Geometry check sheet. Reference: the model listing, model coordinates, mm. A direction names the side the tool comes from. Round coordinates to 2 decimals unless told otherwise and drop trailing zeros. Write each loop counter-clockwise with the first axis right and the second up, starting at its lowest first coordinate (ties: lowest second). Pieces come first, ordered by that corner, then holes.
Item 1: Cross-section at B-B (y = 50). Enter the section's corners in (x, z), then the cut area to 3 significant figures.
Item 2: Draft check along Y on faces 5 (the face through (-21, 0, 0)), 6 (the face through (3.5, 173, 6)), 7 (the face through (-16, 85, 6)), 8 (the face through (21.3, 2.85, 0.92)). Enter one of: pulls with the +Y half, pulls with the -Y half, needs draft (parallel to the pull), parting line crosses it, or undercut.
Item 3: Scan lines: probe 1 along Y at (x, z) = (-19.5, 0); probe 2 along Z at (x, y) = (-20.25, 25); probe 3 along Y at (x, z) = (22.25, 0). Record each from-to range of solid material in increasing order.
Item 4: Cross-section at A-A (y = 7). Enter the section's corners in (x, z).
Item 5: Access from +Z, -Z, +X, -X, +Y, -Y to the whole of each face (thin tool, end or side, straight path). Record for faces 1 (the face through (-17.6, 20, 0)), 2 (the face through (-21, 40, -4)), 3 (the face through (-0.751, 249.86, 3.615)), 4 (the face through (16, 85, 6)).
Item 6: Cross-section at C-C (x = 0). Enter the section's corners in (y, z).
Item 7: Cross-section at D-D (y = 224.5). Enter the section's corners in (x, z), then the cut area to 3 significant figures.
Item 8: Depth check by flat-ended pin: P1, Ø7.5, axis at y = 7, z = 0, coming from the +X side; P2, Ø2, axis at y = 219, z = 6, coming from the -X side; P3, Ø9, axis at x = 6, z = 7, coming from the -Y side; P4, Ø6, axis at x = 23, z = 0, coming from the +Y side. Enter the tip coordinate at first touch or a pass-through.
from build123d import *

# Parameters (mm, degrees)
BOSS_EXTRUDE4_DEPTH     = 10
CUT_EXTRUDE2_DEPTH      = 262.400095639
CUT_EXTRUDE2_DEPTH_BACK = 262.400095639
SKETCH7_R               = 4.25
CUT_EXTRUDE4_DEPTH      = 262.400095639
CUT_EXTRUDE4_DEPTH_BACK = 262.400095639
SKETCH11_W              = 18.643899753
SKETCH11_H              = 220
CUT_EXTRUDE5_DEPTH      = 262.400095639
CUT_EXTRUDE5_DEPTH_BACK = 20
SKETCH12_R              = 2.5
FILLET3_R               = 3


with BuildPart() as part:
    # Sketch6 → Boss-Extrude4 (new, symmetric)
    with BuildSketch(Plane.XY):
        Polygon((-25.1, 0), (-17.6, 0), (-17.6, 40), (-22.1, 40), (-22.1, 80), (22.1, 80), (22.1, 40), (17.6, 40), (17.6, 0), (25.1, 0), (25.1, 85), (3.5, 85), (3.5, 260), (-3.5, 260), (-3.5, 85), (-25.1, 85), align=None)
    extrude(amount=BOSS_EXTRUDE4_DEPTH, both=True)

    # Sketch7 → Cut-Extrude2 (cut, two sides: drawn at the far end of the back side and taken through both)
    with BuildSketch(Plane(origin=(0, 0, 0), x_dir=(0, 0, -1), z_dir=(1, 0, 0)).offset(-CUT_EXTRUDE2_DEPTH_BACK)):
        with Locations((0, 7)):
            Circle(SKETCH7_R)
        with Locations((0, 25)):
            Circle(SKETCH7_R)
    extrude(amount=CUT_EXTRUDE2_DEPTH + CUT_EXTRUDE2_DEPTH_BACK, mode=Mode.SUBTRACT)

    # Sketch11 → Cut-Extrude4 (cut, two sides: drawn at the far end of the back side and taken through both)
    with BuildSketch(Plane(origin=(0, 0, 0), x_dir=(0, 0, -1), z_dir=(1, 0, 0)).offset(-CUT_EXTRUDE4_DEPTH_BACK)):
        with Locations((7.321949876, 150)):
            Rectangle(SKETCH11_W, SKETCH11_H)
    extrude(amount=CUT_EXTRUDE4_DEPTH + CUT_EXTRUDE4_DEPTH_BACK, mode=Mode.SUBTRACT)

    # Sketch12 → Cut-Extrude5 (cut, two sides: drawn at the far end of the back side and taken through both)
    with BuildSketch(Plane(origin=(0, 260, 0), x_dir=(1, 0, 0), z_dir=(0, 1, 0)).offset(-CUT_EXTRUDE5_DEPTH_BACK)):
        with Locations(Location((0, -6, 0), (0, 0, 90))):
            Circle(SKETCH12_R)
    extrude(amount=CUT_EXTRUDE5_DEPTH + CUT_EXTRUDE5_DEPTH_BACK, mode=Mode.SUBTRACT)

    # Fillet3
    fillet3_edges = [part.edges().sort_by_distance(p)[0] for p in [
        (-23.6, 40, 2),
        (23.6, 40, 2),
        (22.1, 40, 6),
        (22.1, 80, 6),
        (-22.1, 80, 6),
        (-22.1, 40, 6),
        (-3.5, 85, 6),
        (3.5, 85, 6),
    ]]
    fillet(fillet3_edges, radius=FILLET3_R)


solid = part.part
Resolved:
1. outline: (-25.1, 2) - (-22.1, 2) - (-22.1, 10) - (-25.1, 10) - close; (22.1, 2) - (25.1, 2) - (25.1, 10) - (22.1, 10) - close
1. area: 48.0 mm2
2. face 5: pulls with the -Y half
2. face 6: needs draft
2. face 7: pulls with the +Y half
2. face 8: undercut
3. probe 1: y = 0 to 2.75, 11.25 to 20.75, 29.25 to 40.03
3. probe 2: z = -10 to -4.25, 4.25 to 10
3. probe 3: y = 0 to 2.75, 11.25 to 20.75, 29.25 to 40.17
4. outline: (-25.1, -10) - (-17.6, -10) - (-17.6, -4.25) - (-25.1, -4.25) - close; (-25.1, 4.25) - (-17.6, 4.25) - (-17.6, 10) - (-25.1, 10) - close; (17.6, -10) - (25.1, -10) - (25.1, -4.25) - (17.6, -4.25) - close; (17.6, 4.25) - (25.1, 4.25) - (25.1, 10) - (17.6, 10) - close
5. face 1: +Z, -Z, -Y
5. face 2: -Z
5. face 3: +Y
5. face 4: +Z, -Z, +X, +Y
6. outline: (80, 2) - (260, 2) - (260, 3.5) - (240, 3.5) - (240, 8.5) - (260, 8.5) - (260, 10) - (80, 10) - close
7. outline: (-3.5, 2) - (3.5, 2) - (3.5, 10) - (-3.5, 10) - close
7. area: 56.0 mm2
8. P1: passes through
8. P2: stops at x = -3.5
8. P3: stops at y = 80
8. P4: stops at y = 85
